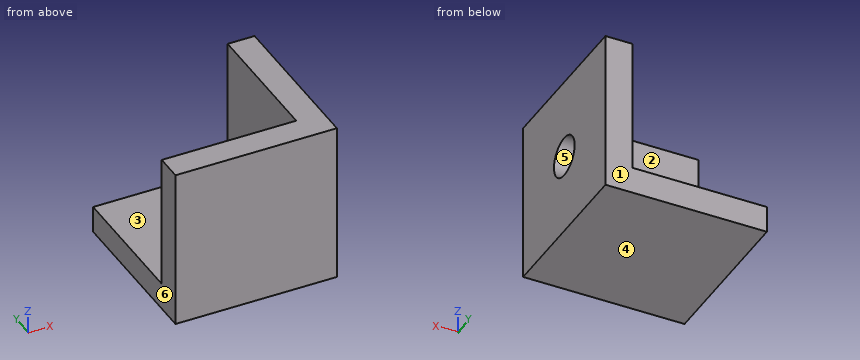
from build123d import *

# Parameters (mm, degrees)
BOSS_EXTRUDE1_DEPTH = 19.05
SKETCH3_W           = 19.05
SKETCH3_H           = 19.05
BOSS_EXTRUDE2_DEPTH = 3.175
SKETCH4_R           = 2.38125
CUT_EXTRUDE1_DEPTH  = 33.995567884


with BuildPart() as part:
    # Sketch2 → Boss-Extrude1 (new body)
    with BuildSketch(Plane(origin=(0, 0, 0), x_dir=(0, 0, -1), z_dir=(1, 0, 0))):
        Polygon((0, 0), (0, 19.05), (-3.175, 19.05), (-3.175, 3.175), (-19.05, 3.175), (-19.05, 0), align=None)
    extrude(amount=BOSS_EXTRUDE1_DEPTH)

    # Sketch3 → Boss-Extrude2 (add)
    with BuildSketch(Plane(origin=(19.05, 0, 0), x_dir=(0, 0, -1), z_dir=(1, 0, 0))):
        with Locations((-9.525, 9.525)):
            Rectangle(SKETCH3_W, SKETCH3_H)
    extrude(amount=-BOSS_EXTRUDE2_DEPTH)

    # Sketch4 → Cut-Extrude1 (cut, through all)
    with BuildSketch(Plane(origin=(19.05, 0, 0), x_dir=(0, 0, -1), z_dir=(1, 0, 0))):
        with Locations((-9.525, 9.525)):
            Circle(SKETCH4_R)
    extrude(amount=-CUT_EXTRUDE1_DEPTH, mode=Mode.SUBTRACT)


solid = part.part
The model under review builds one solid part; all positions refer to its coordinate system, in mm. Face numbers are marked on the shaded views. A direction names the side the tool comes from. Coordinates: 2 decimals unless noted, no trailing zeros. Loops run counter-clockwise (first coordinate to the right, second up) from the corner with the lowest first, then second, coordinate; pieces in that order, holes last. Notation, with made-up numbers: M 20.25,7.5 L 32.25,7.5 A20 ccw 32.25,13.5 Z; hole C 60,-21.5 d4. An arc over 180 degrees is marked long. Put each result on its own line as item: value. Start each with the question number.
Q1. Clearance check with flat-ended pins moving along their axes: pin 1 (2 mm diameter, centred on y = 14.5, z = 7.5, fed in from -X) (3 decimals); pin 2 (10 mm diameter, centred on x = 8.5, z = 15.5, fed in from +Y) (3 decimals); pin 3 (3 mm diameter, centred on y = 9.525, z = 9.525, fed in from -X). State where each tip first meets the part, or that it passes through.
Q2. Add section B-B (y = 8.5). Write out the cut boundary in (x, z) (3 decimals), and give its area (3 significant figures).
Q3. The part is to be moulded in two halves that separate along Z. For the marked faces 3, 4, 5 and 6, say which applies: +Z half, -Z half, draft (parallel to the pull), parting line (faces both ways), or undercut.
Q4. Add section A-A (x = 11.5). Write out the cut boundary in (y, z) (3 decimals).
Q5. For the marked faces 1 and 2, list the 3-axis set-ups (+Z, -Z, +X, -X, +Y, -Y) from which the entire face can be reached by the end or side of a thin tool; tool diameter is ignored.
Q6. Wall thickness on line 1 (X direction, y = 11.5, z = 17.5) (3 decimals); line 2 (Z direction, x = 11, y = 13) (3 decimals): over which ranges is each line inside the solid? List them lowest first.
Q7. Add section C-C (z = 15.25). Write out the cut boundary in (x, y) (3 decimals).
Answers:
1. pin 1: stops at x = 15.875
1. pin 2: stops at y = 3.175
1. pin 3: passes through
2. outline: M 0,0 L 19.05,0 L 19.05,7.376 L 15.875,7.376 L 15.875,3.175 L 0,3.175 Z; M 15.875,11.674 L 19.05,11.674 L 19.05,19.05 L 15.875,19.05 Z
2. area: 97.2 mm^2
3. face 3: +Z half
3. face 4: -Z half
3. face 5: undercut
3. face 6: draft
4. outline: M 0,0 L 19.05,0 L 19.05,3.175 L 3.175,3.175 L 3.175,19.05 L 0,19.05 Z
5. face 1: +Z, -Z, +X, -X, +Y
5. face 2: +Z, -X, +Y
6. line 1: x = 15.875 to 19.05
6. line 2: z = 0 to 3.175
7. outline: M 0,0 L 19.05,0 L 19.05,19.05 L 15.875,19.05 L 15.875,3.175 L 0,3.175 Z
